from build123d import *

# Parameters (mm, degrees)
SKETCH1_R               = 10
BOSS_EXTRUDE1_DEPTH     = 2.5
SKETCH2_R               = 4.5
SKETCH2_R_2             = 2.75
EXTRUDE_THIN1_DEPTH     = 2.5
CUT_EXTRUDE1_DEPTH      = 15.361406616
CUT_EXTRUDE1_DEPTH_BACK = 15.361406616
SKETCH3_R               = 1.55
CUT_EXTRUDE2_START      = -1
SKETCH4_R               = 2.75
CUT_EXTRUDE2_DEPTH      = 1


with BuildPart() as part:
    # Sketch1 → Boss-Extrude1 (new body)
    with BuildSketch(Plane(origin=(0, 0, 0), x_dir=(0, 1, 0), z_dir=(0, 0, 1))):
        with Locations(Location((0, 0, 0), (0, 0, 270))):
            Circle(SKETCH1_R)
    extrude(amount=BOSS_EXTRUDE1_DEPTH)

    # Sketch2 → Extrude-Thin1 (add)
    with BuildSketch(Plane.XY.offset(2.5)):
        Circle(SKETCH2_R)
        Circle(SKETCH2_R_2, mode=Mode.SUBTRACT)
    extrude(amount=EXTRUDE_THIN1_DEPTH)

    # Sketch3 → Cut-Extrude1 (cut, two sides: drawn at the far end of the back side and taken through both)
    with BuildSketch(Plane.XY.offset(2.5).offset(-CUT_EXTRUDE1_DEPTH_BACK)):
        Circle(SKETCH3_R)
        with Locations((7, 0)):
            Circle(SKETCH3_R)
        with Locations((0, 7)):
            Circle(SKETCH3_R)
        with Locations((-7, 0)):
            Circle(SKETCH3_R)
        with Locations((0, -7)):
            Circle(SKETCH3_R)
    extrude(amount=CUT_EXTRUDE1_DEPTH + CUT_EXTRUDE1_DEPTH_BACK, mode=Mode.SUBTRACT)

    # Sketch4 → Cut-Extrude2 (cut)
    with BuildSketch(Plane.XY.offset(2.5).offset(CUT_EXTRUDE2_START)):
        Circle(SKETCH4_R)
    extrude(amount=CUT_EXTRUDE2_DEPTH, mode=Mode.SUBTRACT)


solid = part.part
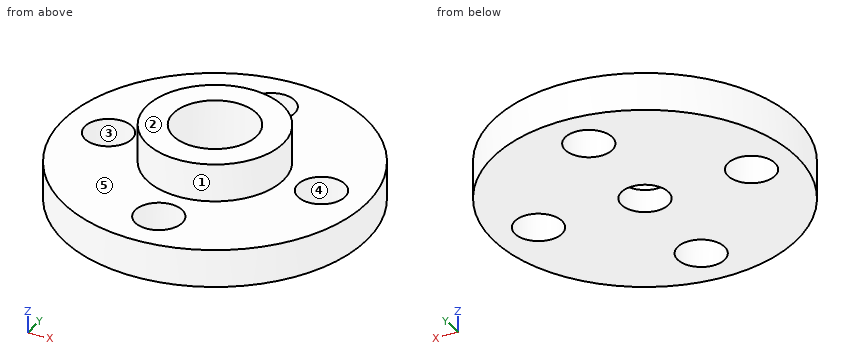
Can you work these out from the model? Positions are in its coordinate system, mm. Face numbers are marked on the shaded views. A direction names the side the tool comes from. Coordinates: 2 decimals unless noted, no trailing zeros. Order: outer loops, then holes, each group sorted by start corner. A loop starts at its lowest first (then second) coordinate and runs counter-clockwise, first axis right, second up. Notation, with made-up numbers: (86, -3.75) -> (122, -3.75) arc R22 ccw to (122, 12.25) -> close; hole circle Ø6 at (-29.75, 64). An arc over 180 degrees is marked (long way). Use one line per item in the form item = value.
Q1. Which directions (+Z, -Z, +X, -X, +Y, -Y) give clear straight access to the entire face, cutting with the end or side of a thin tool? Please do the marked faces 4 and 5.
From the geometry:
face_4 = +Z, -Z
face_5 = +Z
Q2. Imagine slicing it at C-C, the plane z = 2. List the corners of the cut face in (x, y) for me.
From the geometry:
outline = circle Ø20 at (0, 0); hole circle Ø3.1 at (-7, 0); hole circle Ø5.5 at (0, 0); hole circle Ø3.1 at (0, -7); hole circle Ø3.1 at (0, 7); hole circle Ø3.1 at (7, 0)
Q3. Will these pins go through, and if not, where does the flat tip stop? P1, Ø1.5, axis at y = 7.5, z = 1.5, coming from the -X side; P2, Ø8, axis at x = -8, y = 3, coming from the +Z side; P3, Ø1.5, axis at x = -4, z = 3.5, coming from the +Y side; P4, Ø3, axis at x = 7, y = 0, coming from the -Z side.
From the geometry:
P1 = -7.38
P2 = 2.5
P3 = 3.11
P4 = through
Q4. I need wall thicknesses on L1, parallel to Y at x = 0, z = 1; L2, parallel to X at y = -1.25, z = 2.2; L3, parallel to X at y = 0.75, z = 0.2. Which ranges of each line are inside material? Lowest first, please.
From the geometry:
L1 = -10 to -8.55, -5.45 to -1.55, 1.55 to 5.45, 8.55 to 10
L2 = -9.92 to -7.92, -6.08 to -2.45, 2.45 to 6.08, 7.92 to 9.92
L3 = -9.97 to -8.36, -5.64 to -1.36, 1.36 to 5.64, 8.36 to 9.97
Q5. We'd pull the mould along X, two halves only. Please class the marked faces 1, 2 and 3: released by +X, released by -X, zero draft, split by the parting line, or undercut.
From the geometry:
face_1 = split by the parting line
face_2 = zero draft
face_3 = undercut
Q6. Imagine slicing it at A-A, the plane x = 0. List the corners of the cut face in (y, z) for me.
From the geometry:
outline = (-10, 0) -> (-8.55, 0) -> (-8.55, 2.5) -> (-10, 2.5) -> close; (-5.45, 0) -> (-1.55, 0) -> (-1.55, 1.5) -> (-2.75, 1.5) -> (-2.75, 5) -> (-4.5, 5) -> (-4.5, 2.5) -> (-5.45, 2.5) -> close; (1.55, 0) -> (5.45, 0) -> (5.45, 2.5) -> (4.5, 2.5) -> (4.5, 5) -> (2.75, 5) -> (2.75, 1.5) -> (1.55, 1.5) -> close; (8.55, 0) -> (10, 0) -> (10, 2.5) -> (8.55, 2.5) -> close
Q7. Imagine slicing it at D-D, the plane x = -7.75. List the corners of the cut face in (y, z) for me.
From the geometry:
outline = (-6.32, 0) -> (-1.36, 0) -> (-1.36, 2.5) -> (-6.32, 2.5) -> close; (1.36, 0) -> (6.32, 0) -> (6.32, 2.5) -> (1.36, 2.5) -> close
